Here's how the part is built. I have some questions about the finished solid (model axes, mm). A direction names the side the tool comes from. Coordinates: 2 decimals unless noted, no trailing zeros. Loops run counter-clockwise (first coordinate to the right, second up) from the corner with the lowest first, then second, coordinate; pieces in that order, holes last.
from build123d import *

# Parameters (mm, degrees)
F1_DEPTH       = 25
F2_DEPTH       = 10
F3_DEPTH       = 10
F4_DEPTH       = 20
F6_D           = 14.75
F6_CBORE_D     = 22.25
F6_CBORE_DEPTH = 14
F9_SIZE        = 5


with BuildPart() as f1:
    # F0 (on Top) → F1 (new body)
    with BuildSketch(Plane.XY):
        with BuildLine():
            Line((96.5, 100), (-96.5, 100))
            ThreePointArc((-96.5, 100), (-103.5710678119, 97.0710678119), (-106.5, 90))
            Line((-106.5, 90), (-106.5, -90))
            ThreePointArc((-106.5, -90), (-103.5710678119, -97.0710678119), (-96.5, -100))
            Line((-96.5, -100), (-63.5, -100))
            Line((-63.5, -100), (-63.5, -42.2497216032))
            ThreePointArc((-63.5, -42.2497216032), (-58.0047374401, -26.6111405489), (-43.9347826087, -17.8476082112))
            ThreePointArc((-43.9347826087, -17.8476082112), (0.1396103068, 6.3603896932), (24.3476082112, 50.4347826087))
            ThreePointArc((24.3476082112, 50.4347826087), (33.1111405489, 64.5047374401), (48.7497216032, 70))
            Line((48.7497216032, 70), (106.5, 70))
            Line((106.5, 70), (106.5, 90))
            ThreePointArc((106.5, 90), (103.5710678119, 97.0710678119), (96.5, 100))
        make_face()
        with BuildLine():
            ThreePointArc((17.5, 70), (-16.8995859294, 3.7474422497), (-90.8802816901, -6.2320154172))
            ThreePointArc((-90.8802816901, -6.2320154172), (-95.6793281173, -2.5737930287), (-97.5, 3.1793445108))
            Line((-97.5, 3.1793445108), (-97.5, 81))
            ThreePointArc((-97.5, 81), (-94.5710678119, 88.0710678119), (-87.5, 91))
            Line((-87.5, 91), (7.5, 91))
            ThreePointArc((7.5, 91), (14.5710678119, 88.0710678119), (17.5, 81))
            Line((17.5, 81), (17.5, 70))
        make_face(mode=Mode.SUBTRACT)
        with BuildLine():
            Line((106.5, 55), (106.5, 70))
            Line((106.5, 70), (48.7497216032, 70))
            ThreePointArc((48.7497216032, 70), (33.1111405489, 64.5047374401), (24.3476082112, 50.4347826087))
            ThreePointArc((24.3476082112, 50.4347826087), (0.1396103068, 6.3603896932), (-43.9347826087, -17.8476082112))
            ThreePointArc((-43.9347826087, -17.8476082112), (-58.0047374401, -26.6111405489), (-63.5, -42.2497216032))
            Line((-63.5, -42.2497216032), (-63.5, -100))
            Line((-63.5, -100), (-48.5, -100))
            Line((-48.5, -100), (-48.5, -42.2497216032))
            ThreePointArc((-48.5, -42.2497216032), (-46.3018949761, -35.9942891815), (-40.6739130435, -32.4888762464))
            ThreePointArc((-40.6739130435, -32.4888762464), (10.7462120246, -4.2462120246), (38.9888762464, 47.1739130435))
            ThreePointArc((38.9888762464, 47.1739130435), (42.4942891815, 52.8018949761), (48.7497216032, 55))
            Line((48.7497216032, 55), (106.5, 55))
        make_face()
        with BuildLine():
            Line((106.5, -40), (106.5, 55))
            Line((106.5, 55), (48.7497216032, 55))
            ThreePointArc((48.7497216032, 55), (42.4942891815, 52.8018949761), (38.9888762464, 47.1739130435))
            ThreePointArc((38.9888762464, 47.1739130435), (10.7462120246, -4.2462120246), (-40.6739130435, -32.4888762464))
            ThreePointArc((-40.6739130435, -32.4888762464), (-46.3018949761, -35.9942891815), (-48.5, -42.2497216032))
            Line((-48.5, -42.2497216032), (-48.5, -100))
            Line((-48.5, -100), (46.5, -100))
            Line((46.5, -100), (46.5, -55))
            ThreePointArc((46.5, -55), (50.8933982822, -44.3933982822), (61.5, -40))
            Line((61.5, -40), (106.5, -40))
        make_face()
        with BuildLine():
            Line((87.5, -31), (61.5, -31))
            ThreePointArc((61.5, -31), (44.5294372515, -38.0294372515), (37.5, -55))
            Line((37.5, -55), (37.5, -81))
            ThreePointArc((37.5, -81), (34.5710678119, -88.0710678119), (27.5, -91))
            Line((27.5, -91), (-29.5, -91))
            ThreePointArc((-29.5, -91), (-36.5710678119, -88.0710678119), (-39.5, -81))
            Line((-39.5, -81), (-39.5, -49.2476414861))
            ThreePointArc((-39.5, -49.2476414861), (-37.481834214, -43.2234965193), (-32.2419354839, -39.630896205))
            ThreePointArc((-32.2419354839, -39.630896205), (17.1101730553, -10.6101730553), (46.130896205, 38.7419354839))
            ThreePointArc((46.130896205, 38.7419354839), (49.7234965193, 43.981834214), (55.7476414861, 46))
            Line((55.7476414861, 46), (87.5, 46))
            ThreePointArc((87.5, 46), (94.5710678119, 43.0710678119), (97.5, 36))
            Line((97.5, 36), (97.5, -21))
            ThreePointArc((97.5, -21), (94.5710678119, -28.0710678119), (87.5, -31))
        make_face(mode=Mode.SUBTRACT)
        with BuildLine():
            Line((106.5, -90), (106.5, -40))
            Line((106.5, -40), (61.5, -40))
            ThreePointArc((61.5, -40), (50.8933982822, -44.3933982822), (46.5, -55))
            Line((46.5, -55), (46.5, -100))
            Line((46.5, -100), (96.5, -100))
            ThreePointArc((96.5, -100), (103.5710678119, -97.0710678119), (106.5, -90))
        make_face()
        with BuildLine():
            ThreePointArc((-97.5, 3.1793445108), (-95.6793281173, -2.5737930287), (-90.8802816901, -6.2320154172))
            ThreePointArc((-90.8802816901, -6.2320154172), (-16.8995859294, 3.7474422497), (17.5, 70))
            Line((17.5, 70), (17.5, 81))
            ThreePointArc((17.5, 81), (14.5710678119, 88.0710678119), (7.5, 91))
            Line((7.5, 91), (-87.5, 91))
            ThreePointArc((-87.5, 91), (-94.5710678119, 88.0710678119), (-97.5, 81))
            Line((-97.5, 81), (-97.5, 3.1793445108))
        make_face()
        with BuildLine():
            ThreePointArc((37.5, -55), (44.5294372515, -38.0294372515), (61.5, -31))
            Line((61.5, -31), (87.5, -31))
            ThreePointArc((87.5, -31), (94.5710678119, -28.0710678119), (97.5, -21))
            Line((97.5, -21), (97.5, 36))
            ThreePointArc((97.5, 36), (94.5710678119, 43.0710678119), (87.5, 46))
            Line((87.5, 46), (55.7476414861, 46))
            ThreePointArc((55.7476414861, 46), (49.7234965193, 43.981834214), (46.130896205, 38.7419354839))
            ThreePointArc((46.130896205, 38.7419354839), (17.1101730553, -10.6101730553), (-32.2419354839, -39.630896205))
            ThreePointArc((-32.2419354839, -39.630896205), (-37.481834214, -43.2234965193), (-39.5, -49.2476414861))
            Line((-39.5, -49.2476414861), (-39.5, -81))
            ThreePointArc((-39.5, -81), (-36.5710678119, -88.0710678119), (-29.5, -91))
            Line((-29.5, -91), (27.5, -91))
            ThreePointArc((27.5, -91), (34.5710678119, -88.0710678119), (37.5, -81))
            Line((37.5, -81), (37.5, -55))
        make_face()
    extrude(amount=-F1_DEPTH)

    # F0 (on Top) → F2 (join)
    with BuildSketch(Plane.XY):
        with BuildLine():
            Line((106.5, -90), (106.5, -40))
            Line((106.5, -40), (61.5, -40))
            ThreePointArc((61.5, -40), (50.8933982822, -44.3933982822), (46.5, -55))
            Line((46.5, -55), (46.5, -100))
            Line((46.5, -100), (96.5, -100))
            ThreePointArc((96.5, -100), (103.5710678119, -97.0710678119), (106.5, -90))
        make_face()
    extrude(amount=F2_DEPTH)

    # F0 (on Top) → F3 (join)
    with BuildSketch(Plane.XY):
        with BuildLine():
            ThreePointArc((-97.5, 3.1793445108), (-95.6793281173, -2.5737930287), (-90.8802816901, -6.2320154172))
            ThreePointArc((-90.8802816901, -6.2320154172), (-16.8995859294, 3.7474422497), (17.5, 70))
            Line((17.5, 70), (17.5, 81))
            ThreePointArc((17.5, 81), (14.5710678119, 88.0710678119), (7.5, 91))
            Line((7.5, 91), (-87.5, 91))
            ThreePointArc((-87.5, 91), (-94.5710678119, 88.0710678119), (-97.5, 81))
            Line((-97.5, 81), (-97.5, 3.1793445108))
        make_face()
    extrude(amount=F3_DEPTH)

    # F0 (on Top) → F4 (cut)
    with BuildSketch(Plane.XY):
        with BuildLine():
            ThreePointArc((37.5, -55), (44.5294372515, -38.0294372515), (61.5, -31))
            Line((61.5, -31), (87.5, -31))
            ThreePointArc((87.5, -31), (94.5710678119, -28.0710678119), (97.5, -21))
            Line((97.5, -21), (97.5, 36))
            ThreePointArc((97.5, 36), (94.5710678119, 43.0710678119), (87.5, 46))
            Line((87.5, 46), (55.7476414861, 46))
            ThreePointArc((55.7476414861, 46), (49.7234965193, 43.981834214), (46.130896205, 38.7419354839))
            ThreePointArc((46.130896205, 38.7419354839), (17.1101730553, -10.6101730553), (-32.2419354839, -39.630896205))
            ThreePointArc((-32.2419354839, -39.630896205), (-37.481834214, -43.2234965193), (-39.5, -49.2476414861))
            Line((-39.5, -49.2476414861), (-39.5, -81))
            ThreePointArc((-39.5, -81), (-36.5710678119, -88.0710678119), (-29.5, -91))
            Line((-29.5, -91), (27.5, -91))
            ThreePointArc((27.5, -91), (34.5710678119, -88.0710678119), (37.5, -81))
            Line((37.5, -81), (37.5, -55))
        make_face()
    extrude(amount=-F4_DEPTH, mode=Mode.SUBTRACT)

    # F6 (through all)
    with Locations(Plane.XY.offset(10)):
        with Locations((76.5, -70)):
            CounterBoreHole(F6_D / 2, F6_CBORE_D / 2, F6_CBORE_DEPTH)

    # F8: sweep along a path in F0
    with BuildLine(Plane.XY) as f8_path:
        Line((-48.5, -100), (-48.5, -42.2497216032))
        ThreePointArc((-48.5, -42.2497216032), (-46.3018949761, -35.9942891815), (-40.6739130435, -32.4888762464))
        ThreePointArc((-40.6739130435, -32.4888762464), (10.7462120246, -4.2462120246), (38.9888762464, 47.1739130435))
        ThreePointArc((38.9888762464, 47.1739130435), (42.4942891815, 52.8018949761), (48.7497216032, 55))
        Line((48.7497216032, 55), (106.5, 55))
    # F7 (on face) → F8 (sweep)
    with BuildSketch(Plane.XZ.offset(100)):
        with BuildLine():
            Line((-64, 0), (-49, 0))
            Line((-49, 0), (-49, 22.5))
            ThreePointArc((-49, 22.5), (-56.5, 30), (-64, 22.5))
            Line((-64, 22.5), (-64, 0))
        make_face()
    sweep(path=f8_path.line)

    # F9
    f9_edges = [f1.edges().sort_by_distance(p)[0] for p in [
        (-97.5, 42.089672, 10),
    ]]
    chamfer(f9_edges, length=F9_SIZE)


solid = f1.part
Q1. Please list where these lines run through material, in increasing order: probe 1 along Y at (x, z) = (76, 1); probe 2 along Y at (x, z) = (76.5, -1) (3 decimals); probe 3 along Z at (x, y) = (-21, 7.5).
Q2. Suppose I cut it at B-B on x = 76.5. Write out the boundary of the cut face in (y, z) (3 decimals).
Q3. Suppose I cut it at D-D on y = -45. Write out the boundary of the cut face in (x, z), and give its area (3 significant figures).
Q4. Will these pins go through, and if not, where does the flat tip stop? P1, Ø18, axis at x = 76.5, y = -70, coming from the -Z side; P2, Ø18, axis at y = -76, z = 10.5, coming from the -X side; P3, Ø1, axis at x = -20, z = 17, coming from the -Y side; P4, Ø3, axis at x = 75.5, z = 6.5, coming from the +Y side.
Q5. We'd pull the mould along Y, two halves only. Please class faces 5 (the cylindrical face through (78, 63, 30)), 6 (the cylindrical face through (-58.545, -26.487, 11.092)), 7 (the cylindrical face through (9.8, -4.48, 11.41)): pulls with the +Y half, pulls with the -Y half, needs draft (parallel to the pull), parting line crosses it, or undercut.
Q6. Suppose I cut it at C-C on z = 17.5. Write out the boundary of the cut face in (x, y), and give its area (3 significant figures).
Q7. Suppose I cut it at A-A on y = -70. Write out the boundary of the cut face in (x, z) (3 decimals), and give its area (3 significant figures).
Q8. For faces 1 (the flat face through (78, 70.5, 11)), 2 (the cylindrical face through (-95.73, -2.5, 2.46)), 3 (the flat face through (-1, -91, -10)), 4 (the cylindrical face through (-94.49, 88.15, 2.46)), which set-ups out of +Z, -Z, +X, -X, +Y, -Y let a thin tool reach every point of the face, with its end or its side?
Check values:
1. probe 1: y = -100 to -81.11, -58.89 to -40, 55.5 to 70.5
1. probe 2: y = -100 to -81.125, -58.875 to -31, 46 to 100
1. probe 3: z = -25 to 10
2. outline: (-100, -25) - (-77.375, -25) - (-77.375, -4) - (-81.125, -4) - (-81.125, 10) - (-100, 10) - close; (-62.625, -25) - (100, -25) - (100, 0) - (70.5, 0) - (70.5, 22.5) arc R7.5 ccw to (55.5, 22.5) - (55.5, 0) - (46, 0) - (46, -20) - (-31, -20) - (-31, 0) - (-40, 0) - (-40, 10) - (-58.875, 10) - (-58.875, -4) - (-62.625, -4) - close
3. outline: (-106.5, -25) - (106.5, -25) - (106.5, 10) - (50.32, 10) - (50.32, 0) - (39.68, 0) - (39.68, -20) - (-38.55, -20) - (-38.55, 0) - (-49, 0) - (-49, 22.5) arc R7.5 ccw to (-64, 22.5) - (-64, 0) - (-106.5, 0) - close
3. area: 4,750 mm2
4. P1: stops at z = -25
4. P2: stops at x = -64
4. P3: stops at y = -25.24
4. P4: stops at y = 70.5
5. face 5: parting line crosses it
5. face 6: undercut
5. face 7: pulls with the -Y half
6. outline: (-64, -100) - (-49, -100) - (-49, -42.25) arc R10.5 cw to (-40.78, -32) arc R104.5 ccw to (38.5, 47.28) arc R10.5 cw to (48.75, 55.5) - (106.5, 55.5) - (106.5, 70.5) - (48.75, 70.5) arc R25.5 ccw to (23.86, 50.54) arc R89.5 cw to (-44.04, -17.36) arc R25.5 ccw to (-64, -42.25) - close
6. area: 4,110 mm2
7. outline: (-106.5, -25) - (69.125, -25) - (69.125, -4) - (65.375, -4) - (65.375, 10) - (46.5, 10) - (46.5, 0) - (37.5, 0) - (37.5, -20) - (-39.5, -20) - (-39.5, 0) - (-49, 0) - (-49, 22.5) arc R7.5 ccw to (-64, 22.5) - (-64, 0) - (-106.5, 0) - close; (83.875, -25) - (106.5, -25) - (106.5, 10) - (87.625, 10) - (87.625, -4) - (83.875, -4) - close
7. area: 4,190 mm2
8. face 1: +Z, +X, +Y
8. face 2: +Z, -X, -Y
8. face 3: +Z
8. face 4: +Z, -X, +Y
